Can you work these out from the model? Positions are in its coordinate system, mm. Face numbers are marked on the shaded views. A direction names the side the tool comes from. Coordinates: 2 decimals unless noted, no trailing zeros. Order: outer loops, then holes, each group sorted by start corner. A loop starts at its lowest first (then second) coordinate and runs counter-clockwise, first axis right, second up. Notation, with made-up numbers: (78.25, -37) -> (92.25, -37) arc R19 ccw to (92.25, -15) -> close; hole circle Ø4 at (-38.75, 1.5). An arc over 180 degrees is marked (long way). Return JSON: item names as keys, results as strings. Group by question number.
1) For pin 1 (3 mm diameter, centred on x = 18, z = 4.5, fed in from +Y); pin 2 (2.5 mm diameter, centred on x = 3.5, z = 4.5, fed in from -Y); pin 3 (1.9 mm diameter, centred on x = 17.5, z = 4, fed in from +Y); pin 4 (0.6 mm diameter, centred on y = 3.5, z = 5, fed in from -X), each with a flat end and sliding along its axis, tell me the tip position at first contact or that it passes through.
2) If we section it at D-D, the plane x = 6: Please give me the cut outline in (y, z), then the cut area to 3 significant figures.
3) If we section it at A-A, the plane z = 4: Please give me the cut outline in (x, y), then the cut area to 3 significant figures.
4) For the marked faces 1, 2, 3 and 4, which set-ups out of +Z, -Z, +X, -X, +Y, -Y let a thin tool reach every point of the face, with its end or its side?
5) Thinking about a two-plate mould opening in Z: for the marked faces 5, 6 and 7, which applies, +Z half, -Z half, draft (parallel to the pull), parting line (faces both ways), or undercut?
6) If I drill on probe 1 along X at (y, z) = (0.45, 1.5); probe 2 along X at (y, z) = (1.45, 3.5); probe 3 along Z at (x, y) = (-17.5, 1.35), over which ranges is the centre line in solid material (lowest first)? Write a range as from..to.
7) If we section it at B-B, the plane x = -17.5: Please give me the cut outline in (y, z).
8) If we section it at C-C, the plane z = 1: Please give me the cut outline in (x, y), then the cut area to 3 significant figures.
from build123d import *

# Parameters (mm, degrees)
GRUNDK_RPER_DEPTH         = 8
SKIZZE2_R                 = 1.6
BOHRUNG_BEFESTIGUNG_DEPTH = 23.671568098
VERRUNDUNG1_R             = 0.5


with BuildPart() as part:
    # Skizze1 → Grundkörper (new body)
    with BuildSketch(Plane.XY):
        Polygon((-21, 0), (-12, 0), (-12, 3), (12, 3), (12, 0), (21, 0), (21, 2), (14, 2), (14, 5), (-14, 5), (-14, 2), (-21, 2), align=None)
    extrude(amount=GRUNDK_RPER_DEPTH)

    # Skizze2 → Bohrung_Befestigung (cut, through all)
    with BuildSketch(Plane(origin=(0, 2, 0), x_dir=(1, 0, 0), z_dir=(0, 1, 0))):
        with Locations(Location((-17.5, -4, 0), (0, 0, 180))):
            Circle(SKIZZE2_R)
        with Locations((17.5, -4)):
            Circle(SKIZZE2_R)
    extrude(amount=-BOHRUNG_BEFESTIGUNG_DEPTH, mode=Mode.SUBTRACT)

    # Verrundung1
    verrundung1_edges = [part.edges().sort_by_distance(p)[0] for p in [
        (-17.5, 2, 0),
        (-14, 3.5, 0),
        (0, 5, 0),
        (14, 3.5, 0),
        (17.5, 2, 0),
        (21, 1, 0),
        (-21, 1, 0),
        (-21, 2, 4),
        (-14, 2, 4),
        (-14, 5, 4),
        (14, 5, 4),
        (21, 2, 4),
        (21, 1, 8),
        (17.5, 2, 8),
        (14, 3.5, 8),
        (0, 5, 8),
        (-14, 3.5, 8),
        (-17.5, 2, 8),
        (-21, 1, 8),
    ]]
    fillet(verrundung1_edges, radius=VERRUNDUNG1_R)


solid = part.part
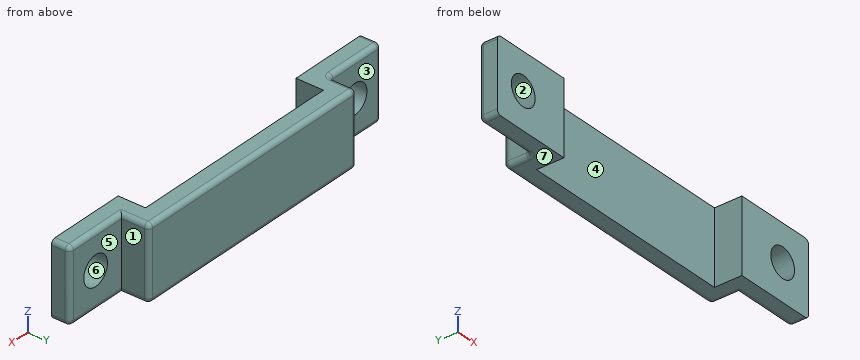
Result sheet:
{
 "1": {"pin 1": "stops at y = 2", "pin 2": "stops at y = 3", "pin 3": "passes through", "pin 4": "stops at x = -14"},
 "2": {"outline": "(3, 0) -> (4.5, 0) arc R0.5 ccw to (5, 0.5) -> (5, 7.5) arc R0.5 ccw to (4.5, 8) -> (3, 8) -> close", "area": "15.9 mm2"},
 "3": {"outline": "(-21, 0) -> (-19.1, 0) -> (-19.1, 2) -> (-20.5, 2) arc R0.5 ccw to (-21, 1.5) -> close; (-15.9, 0) -> (-12, 0) -> (-12, 3) -> (12, 3) -> (12, 0) -> (15.9, 0) -> (15.9, 2) -> (14, 2) -> (14, 4.5) arc R0.5 ccw to (13.5, 5) -> (-13.5, 5) arc R0.5 ccw to (-14, 4.5) -> (-14, 2.5) arc R0.5 cw to (-14.5, 2) -> (-15.9, 2) -> close; (19.1, 0) -> (21, 0) -> (21, 1.5) arc R0.5 ccw to (20.5, 2) -> (19.1, 2) -> close", "area": "83.0 mm2"},
 "4": {"face 1": "+Z, -Z, +X, +Y", "face 2": "+Y, -Y", "face 3": "+Z, -Z, -X, +Y", "face 4": "+Z, -Z, -Y"},
 "5": {"face 5": "draft", "face 6": "undercut", "face 7": "-Z half"},
 "6": {"probe 1": "x = -21..-12, 12..21", "probe 2": "x = -21..-19.02, -15.98..-12, 12..15.98, 19.02..21", "probe 3": "z = 0..2.4, 5.6..8"},
 "7": {"outline": "(0, 0) -> (1.5, 0) arc R0.5 ccw to (2, 0.5) -> (2, 2.4) -> (0, 2.4) -> close; (0, 5.6) -> (2, 5.6) -> (2, 7.5) arc R0.5 ccw to (1.5, 8) -> (0, 8) -> close"},
 "8": {"outline": "(-21, 0) -> (-12, 0) -> (-12, 3) -> (12, 3) -> (12, 0) -> (21, 0) -> (21, 1.5) arc R0.5 ccw to (20.5, 2) -> (14, 2) -> (14, 4.5) arc R0.5 ccw to (13.5, 5) -> (-13.5, 5) arc R0.5 ccw to (-14, 4.5) -> (-14, 2.5) arc R0.5 cw to (-14.5, 2) -> (-20.5, 2) arc R0.5 ccw to (-21, 1.5) -> close", "area": "95.8 mm2"}
}
